```python
from build123d import *

# Parameters (mm, degrees)
F0_R     = 50
F0_R_2   = 12.5
F1_DEPTH = 10
F2_DEPTH = 8
F3_R     = 5
F3_R_2   = 1.25
F4_DEPTH = 25
F5_SIZE  = 1
F6_SIZE  = 0.5


with BuildPart() as f1:
    # F0 (on Top) → F1 (new body)
    with BuildSketch(Plane.XY):
        Circle(F0_R)
        Circle(F0_R_2, mode=Mode.SUBTRACT)
    extrude(amount=F1_DEPTH)

    # F0 (on Top) → F2 (join)
    with BuildSketch(Plane.XY):
        Circle(F0_R_2)
    extrude(amount=F2_DEPTH)

    # F3 (on face) → F4 (cut)
    with BuildSketch(Plane.XY.offset(8)):
        Circle(F3_R)
        with Locations((-7.5, 0)):
            Circle(F3_R_2)
        with Locations((0, 7.5)):
            Circle(F3_R_2)
        with Locations((7.5, 0)):
            Circle(F3_R_2)
        with Locations((0, -7.5)):
            Circle(F3_R_2)
    extrude(amount=-F4_DEPTH, mode=Mode.SUBTRACT)

    # F5
    f5_edges = [f1.edges().sort_by_distance(p)[0] for p in [
        (-50, 0, 0),
        (-50, 0, 10),
    ]]
    chamfer(f5_edges, length=F5_SIZE)

    # F6
    f6_edges = [f1.edges().sort_by_distance(p)[0] for p in [
        (-8.75, 0, 0),
        (-1.25, -7.5, 0),
        (6.25, 0, 0),
        (-1.25, 7.5, 0),
        (6.25, 0, 8),
        (-1.25, -7.5, 8),
        (-1.25, 7.5, 8),
        (-8.75, 0, 8),
    ]]
    chamfer(f6_edges, length=F6_SIZE)


solid = f1.part
```
For this review, take the finished solid that the model builds, in its own axes (mm). Give positions to 0.01 mm unless a question says otherwise; leave off trailing zeros. Write each loop counter-clockwise with the first axis right and the second up, starting at its lowest first coordinate (ties: lowest second). Pieces come first, ordered by that corner, then holes. Notation, with made-up numbers: M 29.25,-16 L 79.25,-16 A20 ccw 79.25,5 Z; hole C 62.5,23.25 d9. An arc over 180 degrees is marked long. Answer as a JSON object with one key per item and string values. Group by question number.
Item 1: Draft analysis for pull direction X (two halves, no side actions). For faces 1 (the flat face through (-0.2, -5.4, 8)), 2 (the cylindrical face through (47.69, 15.02, 4.94)), 3 (the flat face through (10, -10, 10)), state which applies: +X half, -X half, draft (parallel to the pull), parting line (faces both ways), or undercut.
Item 2: Consider section A-A on x = 0. Count the separate pieces of the cut face and the enclosed holes in it, plus the area to 3 significant figures.
Item 3: For probe 1 along Y at (x, z) = (0, 2); probe 2 along Y at (x, z) = (-1, 4.5); probe 3 along Y at (x, z) = (7.5, 5), list the stretches that pass through material, from the lowest coordinate up. Write a range as [from, to].
Item 4: Consider section C-C on z = 3. Write out the cut boundary in (x, y), plus the area to 3 significant figures.
Item 5: For pin 1 Ø4 at (x, y) = (0, -7.5) entering from +Z; pin 2 Ø3 at (x, z) = (26, 6) entering from -Y; pin 3 Ø1 at (y, z) = (-29, 2.5) entering from +X, all flat-tipped, find the tip position at first contact; note any pin that passes through.
Check result:
{
 "1": {"face 1": "undercut", "face 2": "parting line", "face 3": "draft"},
 "2": {"separate pieces": "4", "enclosed holes": "0", "area": "827 mm^2"},
 "3": {"probe 1": "y = [-50, -8.75], [-6.25, -5], [5, 6.25], [8.75, 50]", "probe 2": "y = [-49.99, -8.25], [-6.75, -4.9], [4.9, 6.75], [8.25, 49.99]", "probe 3": "y = [-49.43, -1.25], [1.25, 49.43]"},
 "4": {"outline": "C 0,0 d100; hole C -7.5,0 d2.5; hole C 0,0 d10; hole C 0,-7.5 d2.5; hole C 0,7.5 d2.5; hole C 7.5,0 d2.5", "area": "7,760 mm^2"},
 "5": {"pin 1": "stops at z = 8", "pin 2": "stops at y = -43.59", "pin 3": "stops at x = 41.08"}
}
